```python
from build123d import *

# Parameters (mm, degrees)
BASE_EXTRUDE_DEPTH = 12.7
CIRPATTERN1_COUNT  = 2


with BuildPart() as part:
    # Sketch1 → Base-Extrude (new, symmetric)
    with BuildSketch(Plane.XY):
        with BuildLine():
            Line((-20.6375, 7.9375), (-20.6375, -9.30275))
            ThreePointArc((-20.6375, -9.30275), (-20.33992049, -10.02117049), (-19.6215, -10.31875))
            Line((-19.6215, -10.31875), (-1.016, -10.31875))
            ThreePointArc((-1.016, -10.31875), (-0.29757951, -10.02117049), (0, -9.30275))
            Line((0, -9.30275), (0, 7.9375))
            ThreePointArc((0, 7.9375), (-2.38125, 10.31875), (-4.7625, 7.9375))
            Line((-4.7625, 7.9375), (-3.7465, 7.9375))
            ThreePointArc((-3.7465, 7.9375), (-2.38125, 9.30275), (-1.016, 7.9375))
            Line((-1.016, 7.9375), (-1.016, -9.30275))
            Line((-1.016, -9.30275), (-19.6215, -9.30275))
            Line((-19.6215, -9.30275), (-19.6215, 7.9375))
            ThreePointArc((-19.6215, 7.9375), (-18.25625, 9.30275), (-16.891, 7.9375))
            Line((-16.891, 7.9375), (-15.875, 7.9375))
            ThreePointArc((-15.875, 7.9375), (-18.25625, 10.31875), (-20.6375, 7.9375))
        make_face()
    base_extrude = extrude(amount=BASE_EXTRUDE_DEPTH, both=True)

    # CirPattern1: Base-Extrude ×2 about axis
    cirpattern1_axis = Axis((0, 0, 0), (0, 0, 1))
    for i in range(1, CIRPATTERN1_COUNT):
        add(base_extrude.rotate(cirpattern1_axis, i * 360 / CIRPATTERN1_COUNT))


solid = part.part
```
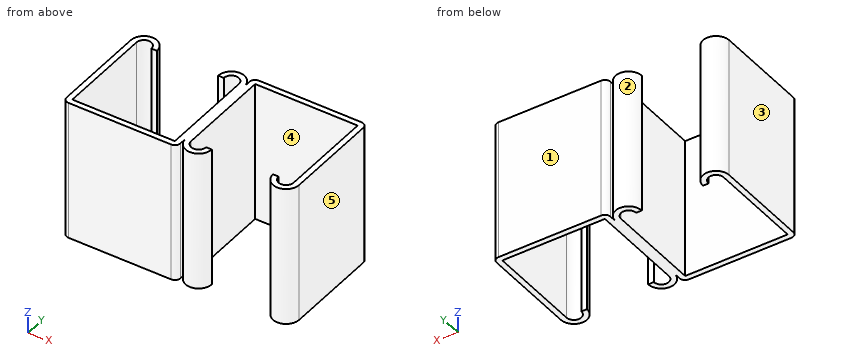
Input: part model. Units: mm. Frame: model coordinates. Face numbers are marked on the shaded views. A direction names the side the tool comes from. Coordinates: 2 decimals unless noted, no trailing zeros. Loops run counter-clockwise (first coordinate to the right, second up) from the corner with the lowest first, then second, coordinate; pieces in that order, holes last. Notation, with made-up numbers: M -24,41.25 L -18,41.25 A14 cw -18,51.25 Z; hole C -2,-33 d4. An arc over 180 degrees is marked long. Use a Markdown table: item, result. Add a question column.
1) Section A-A, the plane y = -3. Return the cut outline in (x, z), plus the area to 3 significant figures.
2) Set-up query: the marked faces 4 and 5. Return all of +Z, -Z, +X, -X, +Y, -Y with unobstructed straight access to the full face (end or side cutting, diameter ignored); none if empty.
3) Line query: L1, parallel to X at y = -4.5, z = 11; L2, parallel to Y at x = 11.5, z = 2.25; L3, parallel to Y at x = -9, z = 3. Output: solid intervals per line, ascending. Write a range as from..to.
4) Section B-B, the plane z = 5.75. Return the cut outline in (x, y) (1 decimal).
5) Pin query (flat end, axial travel): P1, Ø5.5, axis at x = 6, z = -0.5, coming from the -Y side; P2, Ø4, axis at x = -3.5, y = -4.5, coming from the +Z side. Return the tip coordinate at first contact, or that it passes through.
6) Draft query along X for the marked faces 1, 2 and 3. Return one class per face: +X half, -X half, draft (parallel to the pull), parting line (faces both ways), or undercut.
7) Section C-C, the plane x = 11. Return the cut outline in (y, z).
Answer below:
| question | item | result |
|---|---|---|
| 1 | outline | M -20.64,-12.7 L -19.62,-12.7 L -19.62,12.7 L -20.64,12.7 Z; M -1.02,-12.7 L 1.02,-12.7 L 1.02,12.7 L -1.02,12.7 Z; M 19.62,-12.7 L 20.64,-12.7 L 20.64,12.7 L 19.62,12.7 Z |
| 1 | area | 103 mm2 |
| 2 | face 4 | +Z, -Z |
| 2 | face 5 | +Z, -Z, +X, +Y, -Y |
| 3 | L1 | -20.64..-19.62, -1.02..1.02, 19.62..20.64 |
| 3 | L2 | 9.3..10.32 |
| 3 | L3 | -10.32..-9.3 |
| 4 | outline | M -20.6,-9.3 A1 ccw -19.6,-10.3 L -1,-10.3 A1 ccw 0,-9.3 L 0,-7.9 A2.4 ccw 4.8,-7.9 L 3.7,-7.9 A1.4 cw 1,-7.9 L 1,9.3 L 19.6,9.3 L 19.6,-7.9 A1.4 cw 16.9,-7.9 L 15.9,-7.9 A2.4 ccw 20.6,-7.9 L 20.6,9.3 A1 ccw 19.6,10.3 L 1,10.3 A1 ccw 0,9.3 L 0,7.9 A2.4 ccw -4.8,7.9 L -3.7,7.9 A1.4 cw -1,7.9 L -1,-9.3 L -19.6,-9.3 L -19.6,7.9 A1.4 cw -16.9,7.9 L -15.9,7.9 A2.4 ccw -20.6,7.9 Z |
| 5 | P1 | y = -10.15 |
| 5 | P2 | through |
| 6 | face 1 | draft |
| 6 | face 2 | undercut |
| 6 | face 3 | -X half |
| 7 | outline | M 9.3,-12.7 L 10.32,-12.7 L 10.32,12.7 L 9.3,12.7 Z |
